```python
from build123d import *

# Parameters (mm, degrees)
SKETCH1_W           = 50
SKETCH1_H           = 50
SKETCH1_R           = 6.35
SKETCH1_R_2         = 1.778
BOSS_EXTRUDE1_DEPTH = 3.175
SKETCH2_R           = 2.75
SKETCH2_R_2         = 1.5
BOSS_EXTRUDE2_DEPTH = 30
SKETCH3_W           = 50
SKETCH3_H           = 50
BOSS_EXTRUDE3_DEPTH = 3.175
SKETCH4_R           = 2.75
SKETCH4_R_2         = 1.5
BOSS_EXTRUDE4_DEPTH = 30
SKETCH5_W           = 50
SKETCH5_H           = 20
CUT_EXTRUDE1_DEPTH  = 10
FILLET1_R           = 5


with BuildPart() as part:
    # Sketch1 → Boss-Extrude1 (new body)
    with BuildSketch(Plane(origin=(0, 0, 0), x_dir=(1, 0, 0), z_dir=(0, 1, 0))):
        Rectangle(SKETCH1_W, SKETCH1_H)
        Circle(SKETCH1_R, mode=Mode.SUBTRACT)
        with Locations((-9.779, 0)):
            Circle(SKETCH1_R_2, mode=Mode.SUBTRACT)
        with Locations((9.779, 0)):
            Circle(SKETCH1_R_2, mode=Mode.SUBTRACT)
        with Locations((0, 9.779)):
            Circle(SKETCH1_R_2, mode=Mode.SUBTRACT)
        with Locations((0, -9.779)):
            Circle(SKETCH1_R_2, mode=Mode.SUBTRACT)
    extrude(amount=BOSS_EXTRUDE1_DEPTH)

    # Sketch2 → Boss-Extrude2 (add)
    with BuildSketch(Plane(origin=(0, 3.175, 0), x_dir=(1, 0, 0), z_dir=(0, 1, 0))):
        with Locations((20, -20)):
            Circle(SKETCH2_R)
        with Locations((20, -20)):
            Circle(SKETCH2_R_2, mode=Mode.SUBTRACT)
        with Locations((-20, -20)):
            Circle(SKETCH2_R)
        with Locations((-20, -20)):
            Circle(SKETCH2_R_2, mode=Mode.SUBTRACT)
        with Locations((-20, 20)):
            Circle(SKETCH2_R)
        with Locations((-20, 20)):
            Circle(SKETCH2_R_2, mode=Mode.SUBTRACT)
        with Locations((20, 20)):
            Circle(SKETCH2_R)
        with Locations((20, 20)):
            Circle(SKETCH2_R_2, mode=Mode.SUBTRACT)
    extrude(amount=BOSS_EXTRUDE2_DEPTH)

    # Sketch3 → Boss-Extrude3 (add)
    with BuildSketch(Plane(origin=(0, 0, 0), x_dir=(1, 0, 0), z_dir=(0, 1, 0))):
        with Locations((-50, 0)):
            Rectangle(SKETCH3_W, SKETCH3_H)
    extrude(amount=BOSS_EXTRUDE3_DEPTH)

    # Sketch4 → Boss-Extrude4 (add)
    with BuildSketch(Plane(origin=(0, 3.175, 0), x_dir=(1, 0, 0), z_dir=(0, 1, 0))):
        with Locations((-70, 20)):
            Circle(SKETCH4_R)
        with Locations((-70, 20)):
            Circle(SKETCH4_R_2, mode=Mode.SUBTRACT)
        with Locations((-70, -20)):
            Circle(SKETCH4_R)
        with Locations((-70, -20)):
            Circle(SKETCH4_R_2, mode=Mode.SUBTRACT)
        with Locations((-30, -20)):
            Circle(SKETCH4_R)
        with Locations((-30, -20)):
            Circle(SKETCH4_R_2, mode=Mode.SUBTRACT)
        with Locations((-30, 20)):
            Circle(SKETCH4_R)
        with Locations((-30, 20)):
            Circle(SKETCH4_R_2, mode=Mode.SUBTRACT)
    extrude(amount=BOSS_EXTRUDE4_DEPTH)

    # Sketch5 → Cut-Extrude1 (cut)
    with BuildSketch(Plane(origin=(0, 3.175, 0), x_dir=(1, 0, 0), z_dir=(0, 1, 0))):
        with Locations((-42.5, 0)):
            Rectangle(SKETCH5_W, SKETCH5_H)
    extrude(amount=-CUT_EXTRUDE1_DEPTH, mode=Mode.SUBTRACT)

    # Fillet1
    fillet1_edges = [part.edges().sort_by_distance(p)[0] for p in [
        (-67.5, 1.5875, 10),
        (-67.5, 1.5875, -10),
        (-17.5, 1.5875, -10),
        (-17.5, 1.5875, 10),
        (-75, 1.5875, 25),
        (-75, 1.5875, -25),
        (25, 1.5875, 25),
        (25, 1.5875, -25),
    ]]
    fillet(fillet1_edges, radius=FILLET1_R)


solid = part.part
```
For this review, take the finished solid that the model builds, in its own axes (mm). A direction names the side the tool comes from. Round coordinates to 2 decimals unless told otherwise and drop trailing zeros. Write each loop counter-clockwise with the first axis right and the second up, starting at its lowest first coordinate (ties: lowest second). Pieces come first, ordered by that corner, then holes.
1) Take a section at D-D on x = 0. Give the boundary of the cut face in (y, z) (3 decimals), then the cut area to 3 significant figures.
Answer below:
outline: (0, -25) - (3.175, -25) - (3.175, -11.557) - (0, -11.557) - close; (0, -8.001) - (3.175, -8.001) - (3.175, -6.35) - (0, -6.35) - close; (0, 6.35) - (3.175, 6.35) - (3.175, 8.001) - (0, 8.001) - close; (0, 11.557) - (3.175, 11.557) - (3.175, 25) - (0, 25) - close
area: 95.8 mm2
2) For line 1 along Z through (x, y) = (-70, 21); line 2 along X through (y, z) = (29.5, 22); line 3 along X through (y, z) = (5, 22.5), list the stretches that pass through material, from the lowest coordinate up.
Answer below:
line 1: z = -22.75 to -21.5, -18.5 to -17.25, 17.25 to 18.5, 21.5 to 22.75
line 2: x = -71.89 to -68.11, -31.89 to -28.11, -21.89 to -18.11, 18.11 to 21.89
line 3: x = -71.15 to -68.85, -31.15 to -28.85, -21.15 to -18.85, 18.85 to 21.15
3) Insertion check: pin 1 Ø1.5 at (x, z) = (20.5, 19.5) entering from +Y (3 decimals); pin 2 Ø12 at (x, y) = (9.5, 23.5) entering from -Z; pin 3 Ø5 at (y, z) = (21.5, -16.5) entering from -X. Each pin has a flat end and moves straight along its axis. Give the tip position at first contact, or say it passes through.
Answer below:
pin 1: stops at y = 3.175
pin 2: passes through
pin 3: stops at x = -72.56
4) Machinability: for faces 4 (the face through (-43, 2, -10)), 5 (the face through (23, 2, -24)), 6 (the face through (18.89, 17.96, -21.01)), which of the approach directions +Z, -Z, +X, -X, +Y, -Y give a long, thin tool a straight path to every point of the face, cutting with its end or side? Answer none if there is none.
Answer below:
face 4: +Y, -Y
face 5: -Z, +X, +Y, -Y
face 6: +Y
5) Take a section at A-A on y = 12. State how many separate pieces and enclosed holes the cut face has, then the cut area to 3 significant figures.
Answer below:
separate pieces: 8
enclosed holes: 8
area: 134 mm2
6) Take a section at C-C on z = 0. Give the boundary of the cut face in (x, y) (3 decimals), then the cut area to 3 significant figures.
Answer below:
outline: (-75, 0) - (-67.5, 0) - (-67.5, 3.175) - (-75, 3.175) - close; (-17.5, 0) - (-11.557, 0) - (-11.557, 3.175) - (-17.5, 3.175) - close; (-8.001, 0) - (-6.35, 0) - (-6.35, 3.175) - (-8.001, 3.175) - close; (6.35, 0) - (8.001, 0) - (8.001, 3.175) - (6.35, 3.175) - close; (11.557, 0) - (25, 0) - (25, 3.175) - (11.557, 3.175) - close
area: 95.8 mm2
7) Take a section at B-B on x = -30. Give the boundary of the cut face in (y, z) (3 decimals).
Answer below:
outline: (0, -25) - (3.175, -25) - (3.175, -22.75) - (33.175, -22.75) - (33.175, -21.5) - (3.175, -21.5) - (3.175, -18.5) - (33.175, -18.5) - (33.175, -17.25) - (3.175, -17.25) - (3.175, -10) - (0, -10) - close; (0, 10) - (3.175, 10) - (3.175, 17.25) - (33.175, 17.25) - (33.175, 18.5) - (3.175, 18.5) - (3.175, 21.5) - (33.175, 21.5) - (33.175, 22.75) - (3.175, 22.75) - (3.175, 25) - (0, 25) - close
8) Mouldability with a two-part tool opening along X and no side actions: class faces 1 (the face through (21.2, 33.175, 21.2)), 2 (the face through (-74, 2, -23)), 3 (the face through (-67.5, 2, 0)) as +X half, -X half, draft (parallel to the pull), parting line (faces both ways), or undercut.
Answer below:
face 1: draft
face 2: -X half
face 3: undercut
